Model file for the job. Use its own axes, mm. Coordinates: 2 decimals unless noted, no trailing zeros. Order: outer loops, then holes, each group sorted by start corner. A loop starts at its lowest first (then second) coordinate and runs counter-clockwise, first axis right, second up.
from build123d import *

# Parameters (mm, degrees)
F1_DEPTH = 2
F2_W     = 48.4285755818
F2_H     = 3
F3_DEPTH = 2
F4_R     = 1.55
F4_W     = 9.9543361962
F4_H     = 2
F4_W_2   = 47.0205396414
F4_H_2   = 3.0802486688
F5_DEPTH = 2
F7_DEPTH = 2
F9_DEPTH = 2


# Not quite as in the source:
# - a feature names something its author has since deleted; it is built from what else it names


with BuildPart() as f1:
    # F0 (on Front) → F1 (new body)
    with BuildSketch(Plane.XZ):
        Polygon((-23.5, 24), (-33.5, 24), (-33.5, -24), (-23.5, -24), (-23.5, -21), (-23.5, 20.9024734795), align=None)
    extrude(amount=F1_DEPTH)



with BuildPart() as f1b:
    # F0 (on Front) → F1, piece 2 (new body)
    with BuildSketch(Plane.XZ):
        Polygon((33.5, 24), (23.5, 24), (23.5, 20.9024734795), (23.5, -21), (23.5, -24), (33.5, -24), align=None)
    extrude(amount=F1_DEPTH)


with BuildPart() as f1_1:
    add(f1.part)

    add(f1b.part)  # F3 merges F1b
    # F2 (on Front) → F3 (join)
    with BuildSketch(Plane.XZ):
        with Locations((-0.0266507268, -22.4803313563)):
            Rectangle(F2_W, F2_H)
    extrude(amount=F3_DEPTH)

    # F4 (on face) → F5 (join)
    with BuildSketch(Plane(origin=(0, 0, -24), x_dir=(1, 0, 0), z_dir=(0, 0, -1))):
        Polygon((-23.5456638038, 0), (-33.5, 0), (-33.5, -30.0217941403), (-23.5456638038, -30.0217941403), (-23.5456638038, -17.091145739), (-23.5456638038, -14.0108970702), align=None)
        with Locations((-28.5089425743, -23.7523894757)):
            Circle(F4_R, mode=Mode.SUBTRACT)
        with Locations((-28.5089425743, -5.0747846253)):
            Circle(F4_R, mode=Mode.SUBTRACT)
        with Locations((-28.5228319019, 1)):
            Rectangle(F4_W, F4_H)
        Polygon((33.5320457816, 2), (23.4748758376, 2), (23.4748758376, -2.9849826824), (23.4748758376, -14.0108970702), (23.4748758376, -17.091145739), (23.4748758376, -30.0217941403), (33.5320457816, -30.0217941403), align=None)
        with Locations((28.699381277, -23.7523894757)):
            Circle(F4_R, mode=Mode.SUBTRACT)
        with Locations((28.699381277, -5.0747846253)):
            Circle(F4_R, mode=Mode.SUBTRACT)
        with Locations((-0.0353939831, -15.5510214046)):
            Rectangle(F4_W_2, F4_H_2)
    extrude(amount=F5_DEPTH)

    # F6 (on face) → F7 (join)
    with BuildSketch(Plane.YZ.offset(33.5320457816)):
        Polygon((-2, 3.3605340868), (-2.2395208944, 0), (15.6041713825, -24), (18.5901388697, -24), align=None)
        Polygon((18.5901388697, -24), (15.6041713825, -24), (17.091145739, -26), (20.0952365994, -26), align=None)
    extrude(amount=F7_DEPTH)

    # F8 (on face) → F9 (join)
    with BuildSketch(Plane(origin=(-33.5, 0, 0), x_dir=(0, -1, 0), z_dir=(-1, 0, 0))):
        Polygon((2, 2.6476460043), (0, 0.0077232947), (0, -3.6399227096), (2, -1), align=None)
        Polygon((0, 0.0077232947), (-18.1882016523, -24), (-15.4247525627, -24), (0, -3.6399227096), align=None)
        Polygon((-18.1882016523, -24), (-19.7033975273, -26), (-16.9399484377, -26), (-15.4247525627, -24), align=None)
    extrude(amount=F9_DEPTH)


solid = f1_1.part
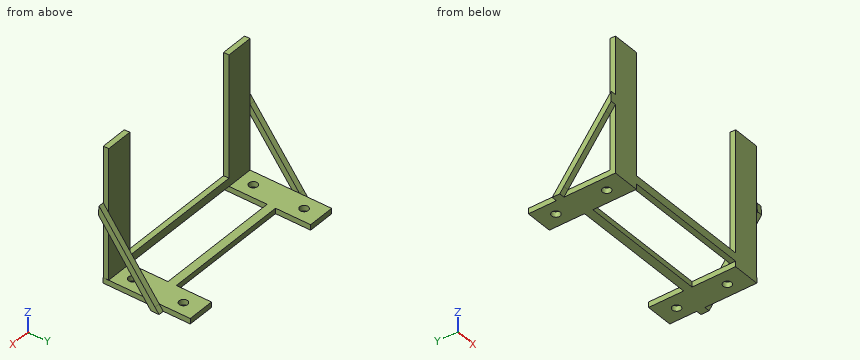
Q1. Cut at D-D, the plane z = -9. List the corners of the cut face in (x, y).
Established:
outline: (-35.5, 4.06) - (-33.5, 4.06) - (-33.5, 6.82) - (-35.5, 6.82) - close; (-33.5, -2) - (-23.5, -2) - (-23.5, 0) - (-33.5, 0) - close; (23.5, -2) - (33.5, -2) - (33.5, 0) - (23.5, 0) - close; (33.53, 4.45) - (35.53, 4.45) - (35.53, 7.3) - (33.53, 7.3) - close
Q2. Probe line 1 (X direction, y = 12.5, z = -18.5); line 2 (Z direction, x = 31, y = 12); line 3 (Y direction, x = -26.5, z = -22). List the from-to ranges inside material, lowest first.
Established:
line 1: x = -35.5 to -33.5, 33.53 to 35.53
line 2: z = -26 to -24
line 3: y = -2 to 0
Q3. Cut at C-C, the plane z = -2.5. List the corners of the cut face in (x, y).
Established:
outline: (-35.5, -0.86) - (-33.5, -0.86) - (-33.5, -2) - (-23.5, -2) - (-23.5, 0) - (-33.5, 0) - (-33.5, 1.9) - (-35.5, 1.9) - close; (23.5, -2) - (33.5, -2) - (33.5, 0) - (23.5, 0) - close; (33.53, -0.38) - (35.53, -0.38) - (35.53, 2.41) - (33.53, 2.41) - close
Q4. Cut at B-B, the plane x = -19. List the corners of the cut face in (y, z), plus the area to 3 significant figures.
Established:
outline: (-2, -23.98) - (0, -23.98) - (0, -20.98) - (-2, -20.98) - close; (14.01, -26) - (17.09, -26) - (17.09, -24) - (14.01, -24) - close
area: 12.2 mm2
Q5. Drop flat-ended pins along their axis: P1, Ø12, axis at y = 5.5, z = 4, coming from the +X side; P2, Ø2, axis at x = -10, y = -1.5, coming from the +Z side; P3, Ø10, axis at x = 6.5, y = 12.5, coming from the +Z side; P4, Ø5.5, axis at y = 3, z = -8.5, coming from the -X side. Give the stop position or say it passes through.
Established:
P1: stops at x = 33.5
P2: stops at z = -20.98
P3: stops at z = -24
P4: stops at x = -35.5
Q6. Cut at A-A, the plane y = 27. List the corners of the cut face in (x, z), plus the area to 3 significant figures.
Established:
outline: (-33.5, -26) - (-23.55, -26) - (-23.55, -24) - (-33.5, -24) - close; (23.47, -26) - (33.53, -26) - (33.53, -24) - (23.47, -24) - close
area: 40.0 mm2
